The model under review builds one solid part; all positions refer to its coordinate system, in mm. A direction names the side the tool comes from. Give positions to 0.01 mm unless a question says otherwise; leave off trailing zeros. Loops run counter-clockwise (first coordinate to the right, second up) from the corner with the lowest first, then second, coordinate; pieces in that order, holes last. Notation, with made-up numbers: M 72.5,66 L 90.5,66 A20 ccw 90.5,89 Z; hole C 43.5,48.5 d3. An arc over 180 degrees is marked long. One line per item, written item: value. Start each with the question number.
Q1. We need section B-B on x = 14. Give the number of separate pieces and of enclosed holes in the cut face, plus the area to 3 significant figures.
Q2. For faces 4 (the face through (7, 0, 12)), 5 (the face through (19, 1, 47.85)), 6 (the face through (18, 1, 15.851)), list the 3-axis set-ups (+Z, -Z, +X, -X, +Y, -Y) from which the entire face can be reached by the end or side of a thin tool; tool diameter is ignored.
Q3. We need section A-A on x = -4. Write out the cut boundary in (y, z).
Q4. For pin 1 (1 mm diameter, centred on x = 19, y = 0.5, fed in from +Z); pin 2 (1 mm diameter, centred on x = 11.5, y = 1, fed in from -Z); pin 3 (1 mm diameter, centred on y = 0.5, z = 50, fed in from -X), all flat-tipped, find the tip position at first contact; note any pin that passes through.
Q5. To check wall thickness, follow line 1 along X through (y, z) = (1, -2); line 2 along Z through (x, y) = (-25, 0.8); line 3 along X through (y, z) = (0.15, 19). State the ranges of each line that lie inside material, in increasing order. Write a range as from..to.
Q6. We need section D-D on z = -26. Write out the cut boundary in (x, y), plus the area to 3 significant figures.
Q7. Mouldability with a two-part tool opening along X and no side actions: class faces 1 (the face through (-7.5, 1, -47)), 2 (the face through (-24, 1, 47.85)), 3 (the face through (-8.53, 1.01, -32.84)) as released by +X, released by -X, zero draft, split by the parting line, or undercut.
```python
from build123d import *

# Parameters (mm, degrees)
EXTRUDE_1_DEPTH          = 2
SKETCH_3_W               = 76.4
SKETCH_3_H               = 2
EXTRUDE_2_DEPTH          = 7
CUT_EXTRUDE_1_DEPTH      = 10
EXTRUDE_4_DEPTH          = 2
PATTERN_LINEAR_2_COUNT   = 2
PATTERN_LINEAR_2_PITCH   = 32
FILLET_3_R               = 0.5
CUT_EXTRUDE_2_DEPTH      = 10
EXTRUDE_5_DEPTH          = 2
CUT_EXTRUDE_3_DEPTH      = 10
CUT_EXTRUDE_4_DEPTH      = 10
FILLET_5_R               = 2
EXTRUDE_9_DEPTH          = 2
FILLET_6_R               = 2
FILLET_7_R               = 1
SKETCH_18_W              = 76.4
SKETCH_18_H              = 2
EXTRUDE_6_DEPTH          = 2
SKETCH_19_W              = 10
SKETCH_19_H              = 10
CUT_EXTRUDE_5_DEPTH      = 3
EXTRUDE_8_DEPTH          = 2
FILLET_8_R               = 2
FILLET_9_R               = 2
SKETCH_21_W              = 3
SKETCH_21_H              = 87.342834434
CUT_EXTRUDE_6_DEPTH      = 3
CUT_EXTRUDE_7_DEPTH      = 1
CUT_EXTRUDE_7_DEPTH_BACK = 3
SKETCH_24_W              = 15
SKETCH_24_H              = 2
EXTRUDE_10_DEPTH         = 3
SKETCH_25_R              = 1
CUT_EXTRUDE_8_DEPTH      = 3


with BuildPart() as part:
    # 草图1 → 凸台-拉伸1 (new body)
    with BuildSketch(Plane(origin=(0, 0, 0), x_dir=(1, 0, 0), z_dir=(0, 1, 0))):
        with BuildLine():
            Line((-38.2, -42.69), (-38.2, -45.85))
            Line((-38.2, -45.85), (38.2, -45.85))
            Line((38.2, -45.85), (38.2, 45.85))
            Line((38.2, 45.85), (-38.2, 45.85))
            Line((-38.2, 45.85), (-38.2, 37.31))
            ThreePointArc((-38.2, 37.31), (1.8, -2.69), (-38.2, -42.69))
        make_face()
    extrude(amount=EXTRUDE_1_DEPTH)

    # 草图3 → 凸台-拉伸2 (add)
    with BuildSketch(Plane(origin=(0, 0, -45.85), x_dir=(-1, 0, 0), z_dir=(0, 0, -1))):
        with Locations((0, 1)):
            Rectangle(SKETCH_3_W, SKETCH_3_H)
    extrude(amount=EXTRUDE_2_DEPTH)

    # 草图5 → 切除-拉伸1 (cut)
    with BuildSketch(Plane(origin=(0, 2, 0), x_dir=(1, 0, 0), z_dir=(0, 1, 0))):
        Polygon((-38.2, 51.26), (38.2, 52.85), (-38.2, 52.85), align=None)
    extrude(amount=-CUT_EXTRUDE_1_DEPTH, mode=Mode.SUBTRACT)

    # 草图7 → 凸台-拉伸4 (add)
    with BuildSketch(Plane.XZ):
        Polygon((25.6, -52.587774869), (25.6, -54.754790576), (9.6, -54.754790576), (9.6, -52.254790576), align=None)
    extrude_4 = extrude(amount=-EXTRUDE_4_DEPTH)

    # 阵列(线性)2: 凸台-拉伸4 ×2
    with Locations(*[Vector(-0.999783511, 0, 0.020807013) * (i * PATTERN_LINEAR_2_PITCH) for i in range(1, PATTERN_LINEAR_2_COUNT)]):
        add(extrude_4)

    # 圆角3
    fillet_3_edges = [part.edges().sort_by_distance(p)[0] for p in [
        (25.6, 1, -54.754790576),
        (9.6, 1, -54.754790576),
        (-6.393072342, 1, -54.088966165),
        (-22.393072342, 1, -54.088966165),
    ]]
    fillet(fillet_3_edges, radius=FILLET_3_R)

    # 草图10 → 切除-拉伸2 (cut)
    with BuildSketch(Plane(origin=(0, 2, 0), x_dir=(1, 0, 0), z_dir=(0, 1, 0))):
        Polygon((-38.882265213, 53.905585721), (39.585789662, 55.538625083), (39.585789662, 48.538625083), (-38.2, 46.919784696), (-39.22769149, 52.889737929), align=None)
    extrude(amount=-CUT_EXTRUDE_2_DEPTH, mode=Mode.SUBTRACT)

    # 草图11 → 凸台-拉伸5 (add)
    with BuildSketch(Plane(origin=(0, 2, 0), x_dir=(1, 0, 0), z_dir=(0, 1, 0))):
        Polygon((-38.2, 46.919784696), (38.2, 49.509784696), (38.2, 48.509784696), align=None)
    extrude(amount=-EXTRUDE_5_DEPTH)

    # 草图13 → 切除-拉伸3 (cut)
    with BuildSketch(Plane.XZ):
        Polygon((38.2, -49.509784696), (37.7, -49.492834434), (38.2, 45.85), align=None)
    extrude(amount=-CUT_EXTRUDE_3_DEPTH, mode=Mode.SUBTRACT)

    # 草图16 → 切除-拉伸4 (cut)
    with BuildSketch(Plane.XZ):
        with BuildLine():
            ThreePointArc((-21.63159016, -39.14883119), (-26.948214114, -40.880601492), (-32.438562967, -41.939652064))
            Line((-32.438562967, -41.939652064), (32.727956442, -44.14883119))
            Line((32.727956442, -44.14883119), (32.754177605, -39.14883119))
            Line((32.754177605, -39.14883119), (-21.63159016, -39.14883119))
        make_face()
        with BuildLine():
            ThreePointArc((-6.399232266, -29.14883119), (-9.26951053, -31.777764346), (-12.35622867, -34.14883119))
            Line((-12.35622867, -34.14883119), (32.780398767, -34.14883119))
            Line((32.780398767, -34.14883119), (32.80661993, -29.14883119))
            Line((32.80661993, -29.14883119), (-6.399232266, -29.14883119))
        make_face()
        with BuildLine():
            ThreePointArc((1.145462918, -19.14883119), (-0.38438284, -21.702193399), (-2.079685213, -24.14883119))
            Line((-2.079685213, -24.14883119), (32.832841093, -24.14883119))
            Line((32.832841093, -24.14883119), (32.859062256, -19.14883119))
            Line((32.859062256, -19.14883119), (1.145462918, -19.14883119))
        make_face()
        with BuildLine():
            ThreePointArc((5.214767949, -9.14883119), (4.446089194, -11.673532869), (3.530729255, -14.14883119))
            Line((3.530729255, -14.14883119), (32.885283419, -14.14883119))
            Line((32.885283419, -14.14883119), (32.911504582, -9.14883119))
            Line((32.911504582, -9.14883119), (5.214767949, -9.14883119))
        make_face()
        with BuildLine():
            Line((32.937725745, -4.14883119), (32.963946908, 0.85116881))
            Line((32.963946908, 0.85116881), (6.762414302, 0.85116881))
            ThreePointArc((6.762414302, 0.85116881), (6.58968308, -1.65560578), (6.277301941, -4.14883119))
            Line((6.277301941, -4.14883119), (32.937725745, -4.14883119))
        make_face()
        with BuildLine():
            Line((33.016389234, 10.85116881), (6.053760559, 10.85116881))
            ThreePointArc((6.053760559, 10.85116881), (6.441352349, 8.360067057), (6.688829476, 5.85116881))
            Line((6.688829476, 5.85116881), (32.990168071, 5.85116881))
            Line((32.990168071, 5.85116881), (33.016389234, 10.85116881))
        make_face()
        with BuildLine():
            Line((33.06883156, 20.85116881), (2.97246589, 20.85116881))
            ThreePointArc((2.97246589, 20.85116881), (3.976569254, 18.378754125), (4.832355682, 15.85116881))
            Line((4.832355682, 15.85116881), (33.042610397, 15.85116881))
            Line((33.042610397, 15.85116881), (33.06883156, 20.85116881))
        make_face()
        with BuildLine():
            Line((33.121273886, 30.85116881), (-3.100875064, 30.85116881))
            ThreePointArc((-3.100875064, 30.85116881), (-1.274777634, 28.410185715), (0.381864384, 25.85116881))
            Line((0.381864384, 25.85116881), (33.095052723, 25.85116881))
            Line((33.095052723, 25.85116881), (33.121273886, 30.85116881))
        make_face()
        with BuildLine():
            Line((33.173710083, 40.85), (-14.350169812, 40.85))
            ThreePointArc((-14.350169812, 40.85), (-10.950539992, 38.501547429), (-7.780649528, 35.85116881))
            Line((-7.780649528, 35.85116881), (33.147495049, 35.85116881))
            Line((33.147495049, 35.85116881), (33.173710083, 40.85))
        make_face()
    extrude(amount=-CUT_EXTRUDE_4_DEPTH, mode=Mode.SUBTRACT)

    # 圆角5
    fillet_5_edges = [part.edges().sort_by_distance(p)[0] for p in [
        (-21.63159016, 1, -39.14883119),
        (32.754177605, 1, -39.14883119),
        (32.727956442, 1, -44.14883119),
        (-6.399232266, 1, -29.14883119),
        (32.80661993, 1, -29.14883119),
        (32.780398767, 1, -34.14883119),
        (-2.079685213, 1, -24.14883119),
        (3.530729255, 1, -14.14883119),
        (5.214767949, 1, -9.14883119),
        (32.911504582, 1, -9.14883119),
        (32.885283419, 1, -14.14883119),
        (32.937725745, 1, -4.14883119),
        (6.688829476, 1, 5.85116881),
        (33.016389234, 1, 10.85116881),
        (32.990168071, 1, 5.85116881),
        (4.832355682, 1, 15.85116881),
        (2.97246589, 1, 20.85116881),
        (0.381864384, 1, 25.85116881),
        (-3.100875064, 1, 30.85116881),
        (33.121273886, 1, 30.85116881),
        (-14.350169812, 1, 40.85),
        (33.173710083, 1, 40.85),
    ]]
    fillet(fillet_5_edges, radius=FILLET_5_R)

    # 草图23 → 凸台-拉伸9 (add)
    with BuildSketch(Plane.XZ):
        with BuildLine():
            Line((30.743661638, -39.14883119), (-21.254296123, -39.14883119))
            ThreePointArc((-21.254296123, -39.14883119), (-21.621062836, -39.182748237), (-21.975389905, -39.283349012))
            ThreePointArc((-21.975389905, -39.283349012), (-27.127035015, -40.926389654), (-32.438562967, -41.939652064))
            Line((-32.438562967, -41.939652064), (30.67101495, -44.079099797))
            ThreePointArc((30.67101495, -44.079099797), (32.125051399, -43.521859473), (32.738749569, -42.090736373))
            Line((32.738749569, -42.090736373), (32.743634136, -41.159319511))
            ThreePointArc((32.743634136, -41.159319511), (32.161578532, -39.738330684), (30.743661638, -39.14883119))
        make_face()
    extrude(amount=-EXTRUDE_9_DEPTH)

    # 圆角6
    fillet_6_edges = [part.edges().sort_by_distance(p)[0] for p in [
        (-12.35622867, 1, -34.14883119),
        (1.145462918, 1, -19.14883119),
        (32.859062256, 1, -19.14883119),
        (32.832841093, 1, -24.14883119),
        (6.277301941, 1, -4.14883119),
        (6.762414302, 1, 0.85116881),
        (32.963946908, 1, 0.85116881),
        (6.053760559, 1, 10.85116881),
        (33.06883156, 1, 20.85116881),
        (33.042610397, 1, 15.85116881),
        (33.095052723, 1, 25.85116881),
        (-7.780649528, 1, 35.85116881),
        (33.147495049, 1, 35.85116881),
    ]]
    fillet(fillet_6_edges, radius=FILLET_6_R)

    # 圆角7
    fillet_7_edges = [part.edges().sort_by_distance(p)[0] for p in [
        (-38.2, 1, 42.69),
        (-38.2, 1, -37.31),
        (-38.2, 1, -46.919784696),
    ]]
    fillet(fillet_7_edges, radius=FILLET_7_R)

    # 草图18 → 凸台-拉伸6 (add)
    with BuildSketch(Plane.XY.offset(45.85)):
        with Locations((0, 1)):
            Rectangle(SKETCH_18_W, SKETCH_18_H)
    extrude(amount=EXTRUDE_6_DEPTH)

    # 草图19 → 切除-拉伸5 (cut, through all)
    with BuildSketch(Plane(origin=(0, 2, 0), x_dir=(1, 0, 0), z_dir=(0, 1, 0))):
        with Locations((33.2, -42.85)):
            Rectangle(SKETCH_19_W, SKETCH_19_H)
    extrude(amount=-CUT_EXTRUDE_5_DEPTH, mode=Mode.SUBTRACT)

    # 草图20 → 凸台-拉伸8 (add)
    with BuildSketch(Plane(origin=(0, 2, 0), x_dir=(1, 0, 0), z_dir=(0, 1, 0))):
        Polygon((25.2, -35.85116881), (33.157977385, -35.85116881), (33.157977385, -37.85), (28.2, -40.85), (25.2, -40.85), align=None)
    extrude(amount=-EXTRUDE_8_DEPTH)

    # 圆角8
    fillet_8_edges = [part.edges().sort_by_distance(p)[0] for p in [
        (25.2, 1, 40.85),
        (25.2, 1, 35.85116881),
    ]]
    fillet(fillet_8_edges, radius=FILLET_8_R)

    # 圆角9
    fillet_9_edges = [part.edges().sort_by_distance(p)[0] for p in [
        (33.157977385, 1, 37.85),
        (28.2, 1, 40.85),
    ]]
    fillet(fillet_9_edges, radius=FILLET_9_R)

    # 草图21 → 切除-拉伸6 (cut, through all)
    with BuildSketch(Plane.XZ):
        with Locations((36.658046139, -5.821417217)):
            Rectangle(SKETCH_21_W, SKETCH_21_H)
    extrude(amount=-CUT_EXTRUDE_6_DEPTH, mode=Mode.SUBTRACT)

    # 草图22 → 切除-拉伸7 (cut, two sides)
    with BuildSketch(Plane.XZ) as cut_extrude_7_sk:
        Polygon((-290.579437235, -45.15), (-39.244125604, -45.15), (60.755874396, -45.15), (60.755874396, -51.15), (-39.244125604, -51.15), (-39.244125604, -47.15), (-39.244125604, 204.185311631), (314.77499341, -152.673510404), (63.439681778, -402.008822036), align=None)
    extrude(amount=CUT_EXTRUDE_7_DEPTH, mode=Mode.SUBTRACT)
    extrude(cut_extrude_7_sk.sketch, amount=-CUT_EXTRUDE_7_DEPTH_BACK, mode=Mode.SUBTRACT)

    # 草图24 → 凸台-拉伸10 (add)
    with BuildSketch(Plane(origin=(0, 0, -45.15), x_dir=(-1, 0, 0), z_dir=(0, 0, -1))):
        with Locations((0, 1)):
            Rectangle(SKETCH_24_W, SKETCH_24_H)
    extrude_10 = extrude(amount=EXTRUDE_10_DEPTH)

    # 草图25 → 切除-拉伸8 (cut, through all)
    with BuildSketch(Plane(origin=(0, 2, 0), x_dir=(1, 0, 0), z_dir=(0, 1, 0))):
        with Locations((-8.5, 45.15)):
            Circle(SKETCH_25_R)
        with Locations((8.5, 45.15)):
            Circle(SKETCH_25_R)
    cut_extrude_8 = extrude(amount=-CUT_EXTRUDE_8_DEPTH, mode=Mode.SUBTRACT)

    # 镜向1: 凸台-拉伸10, 切除-拉伸8 across plane
    add(extrude_10.mirror(Plane.XY.offset(1.35)))
    add(cut_extrude_8.mirror(Plane.XY.offset(1.35)), mode=Mode.SUBTRACT)


solid = part.part
```
Solved:
1. separate pieces: 9
1. enclosed holes: 0
1. area: 106 mm2
2. face 4: +Z, -Z, +X, -X, -Y
2. face 5: +Z, +X, +Y, -Y
2. face 6: +Y, -Y
3. outline: M 0,-48.15 L 2,-48.15 L 2,-34.15 L 0,-34.15 Z; M 0,-29.15 L 2,-29.15 L 2,-18.06 L 0,-18.06 Z; M 0,23.44 L 2,23.44 L 2,35.85 L 0,35.85 Z; M 0,40.85 L 2,40.85 L 2,50.85 L 0,50.85 Z
4. pin 1: z = 47.85
4. pin 2: z = -45.15
4. pin 3: x = -7.5
5. line 1: 1.52..6.56, 32.95..35.16
5. line 2: -45.15..-35.07, 40.45..47.85
5. line 3: -1.68..3.94, 33.05..35.16
6. outline: M -10.33,0 L 35.16,0 L 35.16,2 L -10.33,2 Z
6. area: 91.0 mm2
7. face 1: released by -X
7. face 2: zero draft
7. face 3: undercut
